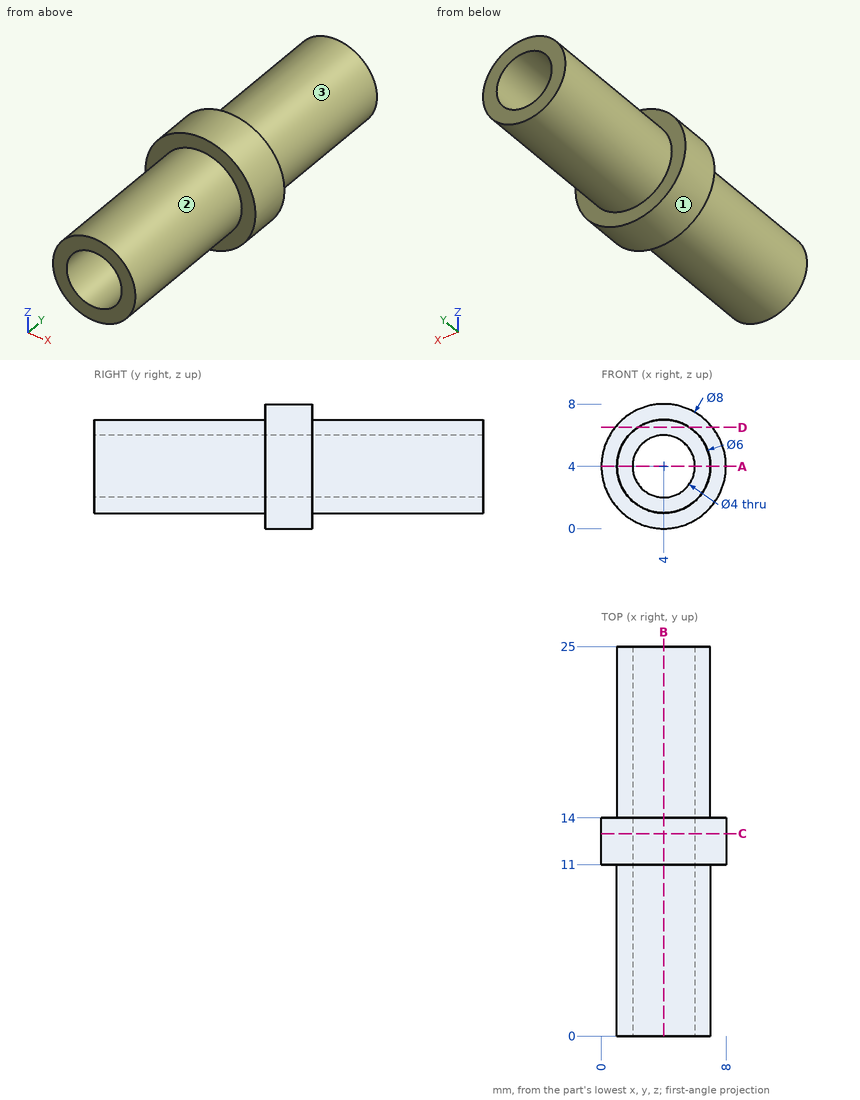
For this review, use the dimensioned drawing (mm, ordinates from the lowest corner) and the shaded views. A direction names the side the tool comes from. Round coordinates to 2 decimals unless told otherwise and drop trailing zeros. Write each loop counter-clockwise with the first axis right and the second up, starting at its lowest first coordinate (ties: lowest second). Pieces come first, ordered by that corner, then holes. Notation, with made-up numbers: (14, 69.5) -> (39, 69.5) arc R12 cw to (39, 78.5) -> close; hole circle Ø2 at (9, 62.25). An arc over 180 degrees is marked (long way). Use CSV: the item, a comma, the result in double quotes.
Q1. For pin 1 Ø1.5 at (x, y) = (6, 21) entering from +Z; pin 2 Ø4 at (x, y) = (1, 20.5) entering from +Z; pin 3 Ø2 at (y, z) = (8, 2.5) entering from -X, all flat-tipped, find the tip position at first contact; note any pin that passes through.
Checks:
pin 1,"z = 6.73"
pin 2,"z = 6.83"
pin 3,"x = 1.04"
Q2. For the marked faces 1, 2 and 3, list the 3-axis set-ups (+Z, -Z, +X, -X, +Y, -Y) from which the entire face can be reached by the end or side of a thin tool; tool diameter is ignored.
Checks:
face 1,"+Y, -Y"
face 2,"-Y"
face 3,"+Y"
Q3. Consider section B-B (x = 4). Give the boundary of the cut face in (y, z).
Checks:
outline,"(0, 1) -> (11, 1) -> (11, 0) -> (14, 0) -> (14, 1) -> (25, 1) -> (25, 2) -> (0, 2) -> close; (0, 6) -> (25, 6) -> (25, 7) -> (14, 7) -> (14, 8) -> (11, 8) -> (11, 7) -> (0, 7) -> close"
Q4. Consider section C-C (y = 13). Give the boundary of the cut face in (x, z).
Checks:
outline,"circle Ø8 at (4, 4); hole circle Ø4 at (4, 4)"
Q5. To check wall thickness, follow probe 1 along Z at (x, y) = (4, 7); probe 2 along Z at (x, y) = (4, 12.25); probe 3 along Y at (x, z) = (2.25, 1.25). State the ranges of each line that lie inside material, in increasing order. Write a range as [from, to].
Checks:
probe 1,"[1, 2], [6, 7]"
probe 2,"[0, 2], [6, 8]"
probe 3,"[11, 14]"
Q6. Consider section A-A (z = 4). Give the boundary of the cut face in (x, y), then the cut area to 3 significant figures.
Checks:
outline,"(0, 11) -> (1, 11) -> (1, 0) -> (2, 0) -> (2, 25) -> (1, 25) -> (1, 14) -> (0, 14) -> close; (6, 0) -> (7, 0) -> (7, 11) -> (8, 11) -> (8, 14) -> (7, 14) -> (7, 25) -> (6, 25) -> close"
area,"56.0 mm²"
Q7. Consider section D-D (z = 6.5). Give the boundary of the cut face in (x, y).
Checks:
outline,"(0.88, 11) -> (2.34, 11) -> (2.34, 0) -> (5.66, 0) -> (5.66, 11) -> (7.12, 11) -> (7.12, 14) -> (5.66, 14) -> (5.66, 25) -> (2.34, 25) -> (2.34, 14) -> (0.88, 14) -> close"
